Check sheet for the modelled part. Datum: model origin and axes. Units: mm. Face numbers are marked on the shaded views. A direction names the side the tool comes from. Round coordinates to 2 decimals unless told otherwise and drop trailing zeros. Write each loop counter-clockwise with the first axis right and the second up, starting at its lowest first coordinate (ties: lowest second). Pieces come first, ordered by that corner, then holes.
Item 1: Cross-section at A-A on x = 0. Enter the section's corners in (y, z).
Item 2: Tool access check on the marked faces 4, 5 and 6. Record the directions out of +Z, -Z, +X, -X, +Y, -Y that give a thin tool (end or side, any length) a straight path to the whole face; none if there is none.
Item 3: Cross-section at D-D on y = -7. Enter the section's corners in (x, z).
Item 4: Material ranges on line 1 (Y direction, x = 12, z = -4.25); line 2 (Y direction, x = 38, z = -8); line 3 (X direction, y = -24, z = -27.5), recorded low to high.
Item 5: Go/stop test with flat-tipped pins: pin 1 Ø6.5 at (x, y) = (-12, -12) entering from +Z; pin 2 Ø1.5 at (x, y) = (3.5, 16) entering from -Z; pin 3 Ø3 at (x, z) = (-5, -26.5) entering from +Y. Record where each tip stops, or that it passes through.
Item 6: Release check for a two-part mould opening along X. For the marked faces 1, 2 and 3 record: +X half, -X half, draft (parallel to the pull), parting line (faces both ways), or undercut.
Item 7: Cross-section at B-B on z = -30. Enter the section's corners in (x, y).
Item 8: Cross-section at C-C on z = -8. Enter the section's corners in (x, y).
from build123d import *

# Parameters (mm, degrees)
SKETCH1_R                 = 13.5
BOSS_EXTRUDE1_DEPTH       = 14
BOSS_EXTRUDE2_START       = -7
SKETCH2_R                 = 13.5
SKETCH2_R_2               = 12.5
BOSS_EXTRUDE2_DEPTH       = 7
SKETCH16_W                = 100
SKETCH16_H                = 35
BOSS_EXTRUDE3_DEPTH       = 8
BOSS_EXTRUDE4_DEPTH       = 8
F_4_0MM_DOWEL_HOLE1_D     = 4
F_4_0MM_DOWEL_HOLE1_DEPTH = 10
F_4_0MM_DOWEL_HOLE1_TIP   = 1.201721238
SKETCH15_R                = 5
CUT_EXTRUDE1_DEPTH        = 78.781745931
CHAMFER1_SIZE             = 10


with BuildPart() as part:
    # Sketch1 → Boss-Extrude1 (new body)
    with BuildSketch(Plane.XY):
        Polygon((-40, -8), (-40, -35), (60, -35), (60, 3.080013472), (60, 22), (-40, 22), align=None)
        Circle(SKETCH1_R, mode=Mode.SUBTRACT)
    extrude(amount=BOSS_EXTRUDE1_DEPTH)

    # Sketch2 → Boss-Extrude2 (add)
    with BuildSketch(Plane.XY.offset(14).offset(BOSS_EXTRUDE2_START)):
        Circle(SKETCH2_R)
        Circle(SKETCH2_R_2, mode=Mode.SUBTRACT)
    extrude(amount=BOSS_EXTRUDE2_DEPTH)

    # Sketch16 → Boss-Extrude3 (add)
    with BuildSketch(Plane.XZ.offset(35)):
        with Locations((10, 17.5)):
            Rectangle(SKETCH16_W, SKETCH16_H)
    extrude(amount=-BOSS_EXTRUDE3_DEPTH)

    # Sketch17 → Boss-Extrude4 (add)
    with BuildSketch(Plane(origin=(60, 0, 0), x_dir=(0, 0, -1), z_dir=(1, 0, 0))):
        Polygon((-34, -27), (-14, 3), (-14, -27), align=None)
    boss_extrude4 = extrude(amount=-BOSS_EXTRUDE4_DEPTH)

    # Mirror1: Boss-Extrude4 across plane
    add(boss_extrude4.mirror(Plane(origin=(10, 0, 0), x_dir=(0, 0, 1), z_dir=(1, 0, 0))))

    # Ø4.0mm Dowel Hole1
    with Locations(Plane(origin=(0, 0, 0), x_dir=(-1, 0, 0), z_dir=(0, 0, -1))):
        with Locations((-12, 12), (12, 12), (12, -12), (-12, -12)):
            Hole(F_4_0MM_DOWEL_HOLE1_D / 2, depth=F_4_0MM_DOWEL_HOLE1_DEPTH)
            with Locations((0, 0, -(F_4_0MM_DOWEL_HOLE1_DEPTH + F_4_0MM_DOWEL_HOLE1_TIP / 2))):  # 118° drill point
                Cone(0, F_4_0MM_DOWEL_HOLE1_D / 2, F_4_0MM_DOWEL_HOLE1_TIP, mode=Mode.SUBTRACT)

    # Sketch15 → Cut-Extrude1 (cut, through all)
    with BuildSketch(Plane(origin=(0, 0, 0), x_dir=(-1, 0, 0), z_dir=(0, 0, -1))):
        with Locations((-38, 0)):
            Circle(SKETCH15_R)
    extrude(amount=-CUT_EXTRUDE1_DEPTH, mode=Mode.SUBTRACT)


with BuildPart() as body_2:
    # Mirror2: mirrored copy
    add(part.part.mirror(Plane.XY))

    # Chamfer1
    chamfer1_edges = [body_2.edges().sort_by_distance(p)[0] for p in [
        (-40, 22, -7),
        (60, 22, -7),
    ]]
    chamfer(chamfer1_edges, length=CHAMFER1_SIZE)


solid = body_2.part
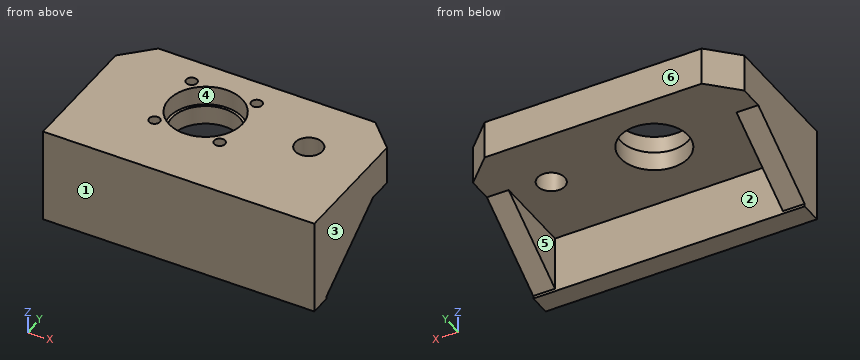
Response values:
1. outline: (-35, -35) - (-27, -35) - (-27, -14) - (-12.5, -14) - (-12.5, -7) - (-13.5, -7) - (-13.5, 0) - (-35, 0) - close; (12.5, -14) - (22, -14) - (22, 0) - (13.5, 0) - (13.5, -7) - (12.5, -7) - close
2. face 4: +Z
2. face 5: -Z, +Y
2. face 6: +Z, -Z, +X, -X, +Y
3. outline: (-40, -20.67) - (-32, -20.67) - (-32, -14) - (-10.36, -14) - (-10.36, -7) - (-11.54, -7) - (-11.54, 0) - (-40, 0) - close; (10.36, -14) - (52, -14) - (52, -20.67) - (60, -20.67) - (60, 0) - (11.54, 0) - (11.54, -7) - (10.36, -7) - close
4. line 1: y = -35 to -14, -10 to -6.18, 6.18 to 10, 14 to 22
4. line 2: y = -35 to -5, 5 to 22
4. line 3: x = -40 to -32, 52 to 60
5. pin 1: stops at z = 0
5. pin 2: stops at z = -14
5. pin 3: stops at y = -27
6. face 1: draft
6. face 2: undercut
6. face 3: +X half
7. outline: (-40, -35) - (60, -35) - (60, -21) - (52, -21) - (52, -27) - (-32, -27) - (-32, -21) - (-40, -21) - close
8. outline: (-40, -35) - (60, -35) - (60, 12) - (50, 22) - (-30, 22) - (-40, 12) - close; hole circle Ø4 at (-12, -12); hole circle Ø4 at (-12, 12); hole circle Ø25 at (0, 0); hole circle Ø4 at (12, -12); hole circle Ø4 at (12, 12); hole circle Ø10 at (38, 0)
